Source: CAD feature listing. Evaluate the final solid. Frame: model axes, mm. A direction names the side the tool comes from. Coordinates: 2 decimals unless noted, no trailing zeros. Write each loop counter-clockwise with the first axis right and the second up, starting at its lowest first coordinate (ties: lowest second). Pieces come first, ordered by that corner, then holes. Notation, with made-up numbers: M 48,48.5 L 56,48.5 A16 ccw 56,79.5 Z; hole C -19,50 d6. An arc over 180 degrees is marked long. One line per item, written item: value. Start each with the question number.
Item 1: Set-up query: faces 4 (the flat face through (-19.525, -7, 0)), 5 (the flat face through (31, -15, 0)), 6 (the flat face through (-42.5, -17, 0)). Return all of +Z, -Z, +X, -X, +Y, -Y with unobstructed straight access to the full face (end or side cutting, diameter ignored); none if empty.
Item 2: Mould query, pull axis Y, two halves, no side actions, for faces 1 (the cylindrical face through (-7.559, -5.796, -0.175)), 2 (the flat face through (19.525, -8, 0)), 3 (the flat face through (-31, -15, 0)). Classes: released by +Y, released by -Y, zero draft, split by the parting line, or undercut.
Item 3: Cut plane A-A, the plane x = 0. Output: boundary loops of the cut face in (y, z) (3 decimals).
Item 4: Cut plane B-B, the plane y = 3. Output: boundary loops of the cut face in (x, z).
Item 5: Cut plane D-D, the plane x = 33. Output: boundary loops of the cut face in (y, z), then the cut area to 3 significant figures.
Item 6: Ray query, L1, parallel to Y at x = 0, z = -5.75 (3 decimals); L2, parallel to X at y = -8, z = -8.75 (3 decimals); L3, parallel to Y at x = 32.5, z = -2. Return the intervals inside material, ascending. Write a range as from..to.
Item 7: Cut plane C-C, the plane z = -8.5. Output: boundary loops of the cut face in (x, y) (3 decimals).
Item 8: Pin query (flat end, axial travel): P1, Ø8, axis at y = -9, z = -8, coming from the +X side (3 decimals); P2, Ø4, axis at y = -10, z = 3, coming from the -X side (3 decimals); P3, Ø11.5, axis at x = 32.5, z = -4, coming from the +Y side. Return the tip coordinate at first contact, or that it passes through.
```python
from build123d import *

# Parameters (mm, degrees)
SKETCH1_R           = 9.525
BOSS_EXTRUDE1_DEPTH = 12.5


with BuildPart() as part:
    # Sketch1 → Boss-Extrude1 (new, symmetric)
    with BuildSketch(Plane.XY):
        with BuildLine():
            Line((-19.525, 0), (-19.525, -15))
            Line((-19.525, -15), (-42.5, -15))
            Line((-42.5, -15), (-42.5, -20))
            Line((-42.5, -20), (42.5, -20))
            Line((42.5, -20), (42.5, -15))
            Line((42.5, -15), (19.525, -15))
            Line((19.525, -15), (19.525, 0))
            ThreePointArc((19.525, 0), (0, 19.525), (-19.525, 0))
        make_face()
        Circle(SKETCH1_R, mode=Mode.SUBTRACT)
    extrude(amount=BOSS_EXTRUDE1_DEPTH, both=True)


solid = part.part
```
From the geometry:
1. face 4: +Z, -Z, -X, +Y
1. face 5: +Z, -Z, +X, +Y
1. face 6: +Z, -Z, -X, +Y, -Y
2. face 1: undercut
2. face 2: zero draft
2. face 3: released by +Y
3. outline: M -20,-12.5 L -9.525,-12.5 L -9.525,12.5 L -20,12.5 Z; M 9.525,-12.5 L 19.525,-12.5 L 19.525,12.5 L 9.525,12.5 Z
4. outline: M -19.29,-12.5 L -9.04,-12.5 L -9.04,12.5 L -19.29,12.5 Z; M 9.04,-12.5 L 19.29,-12.5 L 19.29,12.5 L 9.04,12.5 Z
5. outline: M -20,-12.5 L -15,-12.5 L -15,12.5 L -20,12.5 Z
5. area: 125 mm²
6. L1: y = -20..-9.525, 9.525..19.525
6. L2: x = -19.525..-5.17, 5.17..19.525
6. L3: y = -20..-15
7. outline: M -42.5,-20 L 42.5,-20 L 42.5,-15 L 19.525,-15 L 19.525,0 A19.525 ccw -19.525,0 L -19.525,-15 L -42.5,-15 Z; hole C 0,0 d19.05
8. P1: stops at x = 19.525
8. P2: stops at x = -19.525
8. P3: stops at y = -15
